```python
from build123d import *

# Parameters (mm, degrees)
ESKIZ_KONTUR_R        = 60
ESKIZ_KONTUR_W        = 12.2
ESKIZ_KONTUR_H        = 5.2
ESKIZ_KONTUR_W_2      = 8
ESKIZ_KONTUR_H_2      = 16
PLASTINA_DEPTH        = 5
OTVERSTIYA_DEPTH      = 86
OTVERSTIYA_DEPTH_BACK = 86
ESKIZ_OTVERSTIYA_R    = 1.65
ESKIZ_OTVERSTIYA_R_2  = 2.75


with BuildPart() as part:
    # Eskiz_kontur → Plastina (new body)
    with BuildSketch(Plane.XY):
        Circle(ESKIZ_KONTUR_R)
        with Locations((-29, -37.5)):
            Rectangle(ESKIZ_KONTUR_W, ESKIZ_KONTUR_H, mode=Mode.SUBTRACT)
        with Locations((11, -37.5)):
            Rectangle(ESKIZ_KONTUR_W, ESKIZ_KONTUR_H, mode=Mode.SUBTRACT)
        with Locations((-50, 0)):
            Rectangle(ESKIZ_KONTUR_W_2, ESKIZ_KONTUR_H_2, mode=Mode.SUBTRACT)
        with Locations((-29, 30)):
            Rectangle(ESKIZ_KONTUR_W, ESKIZ_KONTUR_H, mode=Mode.SUBTRACT)
        with Locations((11, 30)):
            Rectangle(ESKIZ_KONTUR_W, ESKIZ_KONTUR_H, mode=Mode.SUBTRACT)
    extrude(amount=PLASTINA_DEPTH)

    # Eskiz_otverstiya → Otverstiya (cut, two sides: drawn at the far end of the back side and taken through both)
    with BuildSketch(Plane.XY.offset(-OTVERSTIYA_DEPTH_BACK)):
        with Locations((-9, -37.5)):
            Circle(ESKIZ_OTVERSTIYA_R)
        with Locations((0, -27)):
            Circle(ESKIZ_OTVERSTIYA_R)
        with Locations((-5.65685, -5.65685)):
            Circle(ESKIZ_OTVERSTIYA_R)
        with Locations((5.65685, -5.65685)):
            Circle(ESKIZ_OTVERSTIYA_R)
        with Locations((-27, 0)):
            Circle(ESKIZ_OTVERSTIYA_R)
        Circle(ESKIZ_OTVERSTIYA_R_2)
        with Locations((-5.65685, 5.65685)):
            Circle(ESKIZ_OTVERSTIYA_R)
        with Locations((5.65685, 5.65685)):
            Circle(ESKIZ_OTVERSTIYA_R)
        with Locations((27, 0)):
            Circle(ESKIZ_OTVERSTIYA_R)
        with Locations((-9, 30)):
            Circle(ESKIZ_OTVERSTIYA_R)
        with Locations((0, 27)):
            Circle(ESKIZ_OTVERSTIYA_R)
    extrude(amount=OTVERSTIYA_DEPTH + OTVERSTIYA_DEPTH_BACK, mode=Mode.SUBTRACT)


solid = part.part
```
Model file for the job. Use its own axes, mm. A direction names the side the tool comes from. Give positions to 0.01 mm unless a question says otherwise; leave off trailing zeros. Order: outer loops, then holes, each group sorted by start corner. A loop starts at its lowest first (then second) coordinate and runs counter-clockwise, first axis right, second up.
1) Saw through at B-B, the plane x = -48.5. Write the cut outline in (y, z).
2) Wall check: probe 1 along Y at (x, z) = (0, 3.95); probe 2 along X at (y, z) = (-4.5, 2.05); probe 3 along X at (y, z) = (30, 3). Give the ranges that are in metal, low to high.
3) Saw through at A-A, the plane y = -37.5. Write the cut outline in (x, z), then the cut area to 3 significant figures.
4) Saw through at C-C, the plane z = 3.5. Count the separate pieces of the cut face and the enclosed holes in it, then the cut area to 3 significant figures.
5) Mould opens along Y. For faces 1 (the flat face through (17.1, -38, 2)), 2 (the flat face through (12, 1, 0)), 3 (the flat face through (-29, -34.9, 2)), 4 (the cylindrical face through (-59.94, 2.64, 2.46)) say: +Y half, -Y half, draft (parallel to the pull), parting line (faces both ways), or undercut.
6) Saw through at D-D, the plane x = -9. Write the cut outline in (y, z).
7) Pin check, flat tips, straight feed: pin 1 (1 mm diameter, centred on x = -30.5, z = 2.5, fed in from -Y); pin 2 (2.5 mm diameter, centred on x = -29, z = 1.5, fed in from -Y); pin 3 (1.5 mm diameter, centred on x = -38.5, z = 3.5, fed in from +Y); pin 4 (3 mm diameter, centred on x = -9, y = -37.5, fed in from -Z). Stop position of each tip, or through.
8) 3-axis set-ups, long thin cutter, end or side, ignore diameter. For faces 5 (the flat face through (-29, 32.6, 2)), 6 (the flat face through (12, 1, 5)): which of +Z, -Z, +X, -X, +Y, -Y reach the whole face in a straight line?
Computed:
1. outline: (-35.32, 0) - (-8, 0) - (-8, 5) - (-35.32, 5) - close; (8, 0) - (35.32, 0) - (35.32, 5) - (8, 5) - close
2. probe 1: y = -60 to -28.65, -25.35 to -2.75, 2.75 to 25.35, 28.65 to 60
2. probe 2: x = -59.83 to -54, -46 to -6.83, -4.48 to 4.48, 6.83 to 59.83
2. probe 3: x = -51.96 to -35.1, -22.9 to -10.65, -7.35 to 4.9, 17.1 to 51.96
3. outline: (-46.84, 0) - (-35.1, 0) - (-35.1, 5) - (-46.84, 5) - close; (-22.9, 0) - (-10.65, 0) - (-10.65, 5) - (-22.9, 5) - close; (-7.35, 0) - (4.9, 0) - (4.9, 5) - (-7.35, 5) - close; (17.1, 0) - (46.84, 0) - (46.84, 5) - (17.1, 5) - close
3. area: 330 mm2
4. separate pieces: 1
4. enclosed holes: 16
4. area: 10,800 mm2
5. face 1: undercut
5. face 2: draft
5. face 3: undercut
5. face 4: parting line
6. outline: (-59.32, 0) - (-39.15, 0) - (-39.15, 5) - (-59.32, 5) - close; (-35.85, 0) - (28.35, 0) - (28.35, 5) - (-35.85, 5) - close; (31.65, 0) - (59.32, 0) - (59.32, 5) - (31.65, 5) - close
7. pin 1: stops at y = -51.96
7. pin 2: stops at y = -53.2
7. pin 3: stops at y = 46.64
7. pin 4: passes through
8. face 5: +Z, -Z
8. face 6: +Z, +X, -X, +Y, -Y
